from build123d import *

# Parameters (mm, degrees)
SKETCH1_R                 = 6.35
SKETCH1_R_2               = 2.5
BOSS_EXTRUDE1_DEPTH       = 6.35
SKETCH2_R                 = 3.175
SKETCH2_R_2               = 2.5
BOSS_EXTRUDE2_DEPTH       = 19.05
F_4_40_TAPPED_HOLE1_D     = 2.2606
F_4_40_TAPPED_HOLE1_DEPTH = 6.349
F_4_40_TAPPED_HOLE1_TIP   = 0.679152758


with BuildPart() as part:
    # Sketch1 → Boss-Extrude1 (new body)
    with BuildSketch(Plane.XY):
        Circle(SKETCH1_R)
        Circle(SKETCH1_R_2, mode=Mode.SUBTRACT)
    extrude(amount=BOSS_EXTRUDE1_DEPTH)

    # Sketch2 → Boss-Extrude2 (add)
    with BuildSketch(Plane.XY.offset(6.35)):
        with Locations(Location((0, 0, 0), (0, 0, 180))):
            Circle(SKETCH2_R)
        Circle(SKETCH2_R_2, mode=Mode.SUBTRACT)
    extrude(amount=BOSS_EXTRUDE2_DEPTH)

    # #4-40 Tapped Hole1
    with Locations(Plane.ZY.offset(6.35)):
        with Locations((3.191608174, 0)):
            Hole(F_4_40_TAPPED_HOLE1_D / 2, depth=F_4_40_TAPPED_HOLE1_DEPTH)
            with Locations((0, 0, -(F_4_40_TAPPED_HOLE1_DEPTH + F_4_40_TAPPED_HOLE1_TIP / 2))):  # 118° drill point
                Cone(0, F_4_40_TAPPED_HOLE1_D / 2, F_4_40_TAPPED_HOLE1_TIP, mode=Mode.SUBTRACT)


solid = part.part
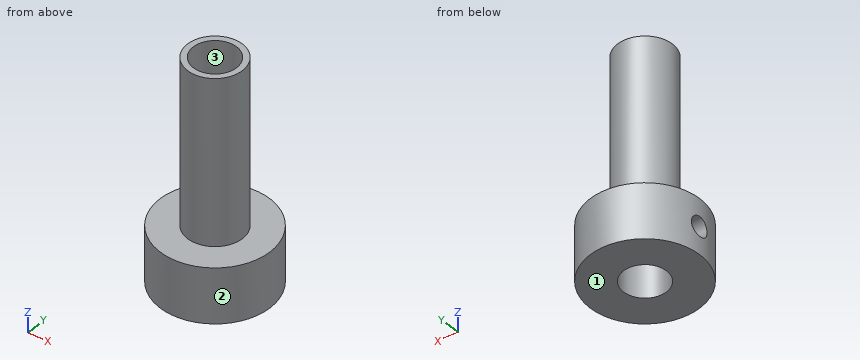
Source: CAD feature listing. Evaluate the final solid. Frame: model axes, mm. Face numbers are marked on the shaded views. Round coordinates to 2 decimals unless told otherwise and drop trailing zeros. Loops run counter-clockwise (first coordinate to the right, second up) from the corner with the lowest first, then second, coordinate; pieces in that order, holes last.
Q1. Mould query, pull axis X, two halves, no side actions, for the marked faces 1, 2 and 3. Classes: pulls with the +X half, pulls with the -X half, needs draft (parallel to the pull), parting line crosses it, or undercut.
Q2. Section B-B, the plane y = 0. Return loops of the section in (x, z) (3 decimals), plus the area to 3 significant figures.
Q3. Section C-C, the plane y = -2. Return loops of the section in (x, z).
Q4. Section D-D, the plane z = 8. Return loops of the section in (x, y) (3 decimals).
Q5. Ray query, line 1 (X direction, y = 0, z = 6.25); line 2 (Y direction, x = 0, z = 6.5) (3 decimals); line 3 (Z direction, x = 2.25, y = 3.5). Return the intervals inside material, ascending.
Q6. First-contact query: P1, Ø2, axis at y = 1.5, z = 12.5, coming from the +X side; P2, Ø3, axis at y = 0, z = 3.19, coming from the -X side; P3, Ø6, axis at y = -3.5, z = 5, coming from the +X side; P4, Ø3, axis at x = 0, y = 0, coming from the +Z side. Flat tips, straight axial feed; report the tip coordinate or a pass-through.
Q7. Section A-A, the plane x = 0. Return loops of the section in (y, z) (3 decimals).
Solutions:
1. face 1: needs draft
1. face 2: parting line crosses it
1. face 3: undercut
2. outline: (-6.35, 0) - (-2.5, 0) - (-2.5, 2.061) - (-6.35, 2.061) - close; (-6.35, 4.322) - (-2.5, 4.322) - (-2.5, 25.4) - (-3.175, 25.4) - (-3.175, 6.35) - (-6.35, 6.35) - close; (2.5, 0) - (6.35, 0) - (6.35, 6.35) - (3.175, 6.35) - (3.175, 25.4) - (2.5, 25.4) - close
2. area: 65.9 mm2
3. outline: (-6.03, 0) - (-1.5, 0) - (-1.5, 25.4) - (-2.47, 25.4) - (-2.47, 6.35) - (-6.03, 6.35) - close; (1.5, 0) - (6.03, 0) - (6.03, 6.35) - (2.47, 6.35) - (2.47, 25.4) - (1.5, 25.4) - close
4. outline: circle Ø6.35 at (0, 0); hole circle Ø5 at (0, 0)
5. line 1: x = -6.35 to -2.5, 2.5 to 6.35
5. line 2: y = -3.175 to -2.5, 2.5 to 3.175
5. line 3: z = 0 to 6.35
6. P1: stops at x = 3.14
6. P2: stops at x = -6.35
6. P3: stops at x = 6.33
6. P4: passes through
7. outline: (-6.35, 0) - (-2.5, 0) - (-2.5, 25.4) - (-3.175, 25.4) - (-3.175, 6.35) - (-6.35, 6.35) - close; (2.5, 0) - (6.35, 0) - (6.35, 6.35) - (3.175, 6.35) - (3.175, 25.4) - (2.5, 25.4) - close
